Input: part model. Units: mm. Frame: model coordinates. Face numbers are marked on the shaded views. A direction names the side the tool comes from. Coordinates: 2 decimals unless noted, no trailing zeros. Write each loop counter-clockwise with the first axis right and the second up, starting at its lowest first coordinate (ties: lowest second). Pieces come first, ordered by that corner, then holes.
Autodesk Inventor part; units mm, degrees
ref_plane "YZ Plane" through (0, 0, 0) normal (1, 0, 0) x (0, 1, 0)
ref_plane "XZ Plane" through (0, 0, 0) normal (0, 1, 0) x (-1, 0, 0)
ref_plane "XY Plane" through (0, 0, 0) normal (0, 0, 1) x (1, 0, 0)
sketch "Boceto1" plane through (0, 0, 0) normal (0, 0, 1) x (1, 0, 0)
  arc A0 (30, 0) -> (-30, 0) centre (0, 0) ccw
  line L0 (5, 0) -> (30, 0)
  arc A1 (-30, 0) -> (30, 0) centre (0, 0) ccw
  circle A2 centre (0, 0) radius 5
  line L1 (0, 0) -> (0, 12.5)
  line L2 (0, 12.5) -> (-12.5, 12.5)
  line L3 (-12.5, 12.5) -> (-12.5, 16.7)
  line L4 (-12.5, 16.7) -> (12.5, 16.7)
  line L5 (12.5, 16.7) -> (12.5, 12.5)
  line L6 (12.5, 12.5) -> (0, 12.5)
  line L7 (0, 0) -> (0, -12.5)
  line L8 (0, -12.5) -> (-12.5, -12.5)
  line L9 (-12.5, -12.5) -> (-12.5, -16.7)
  line L10 (-12.5, -16.7) -> (12.5, -16.7)
  line L11 (12.5, -16.7) -> (12.5, -12.5)
  line L12 (0, -12.5) -> (12.5, -12.5)
  point P0 (0.3554, 29.9979)
  point P1 (0.3554, -29.9979)
  point P2 (-5, 0)
  dimension "d0" = 60
  dimension "d13" = 10
  dimension "d14" = 12.5
  dimension "d15" = 12.5
  dimension "d16" = 4.2
  dimension "d17" = 25
  dimension "d18" = 12.5
  dimension "d19" = 12.5
  dimension "d20" = 4.2
  dimension "d21" = 25
extrude "Extrusión2" add sketch "Boceto1" along normal blind 8
properties part number "leva00" material "Madera (abedul)"
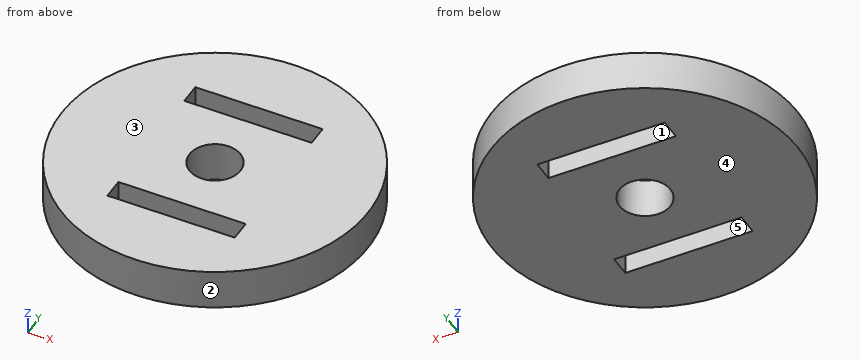
Item 1: Section query A-A, the plane x = 0. Return loops of the section in (y, z), then the cut area to 3 significant figures.
Item 2: Section query B-B, the plane z = 6.5. Return loops of the section in (x, y).
Item 3: Material intervals for line 1 (Y direction, x = 0, z = 5.5); line 2 (X direction, y = 0, z = 4.5); line 3 (Y direction, x = -9, z = 3.5), sorted ascending.
Item 4: Pin query (flat end, axial travel): pin 1 Ø2 at (y, z) = (13.5, 4.5) entering from -X; pin 2 Ø4.5 at (y, z) = (-14, 3.5) entering from +X; pin 3 Ø1 at (x, z) = (16.5, 3.5) entering from -Y. Return the tip coordinate at first contact, or that it passes through.
Item 5: Section query D-D, the plane x = 9. Return loops of the section in (y, z), then the cut area to 3 significant figures.
Item 6: Section query C-C, the plane y = 2. Return loops of the section in (x, z).
Item 7: Pull-direction query (X, two-part tool) for the marked faces 1, 2 and 3; classes: released by +X, released by -X, zero draft, split by the parting line, or undercut.
Item 8: Access query for the marked faces 4 and 5. Directions: +Z, -Z, +X, -X, +Y, -Y. A direction counts if a zero-diameter tool reaches every point of the face in a straight line with its end or side. Return the directions, or none.
The answers:
1. outline: (-30, 0) - (-16.7, 0) - (-16.7, 8) - (-30, 8) - close; (-12.5, 0) - (-5, 0) - (-5, 8) - (-12.5, 8) - close; (5, 0) - (12.5, 0) - (12.5, 8) - (5, 8) - close; (16.7, 0) - (30, 0) - (30, 8) - (16.7, 8) - close
1. area: 333 mm2
2. outline: circle Ø60 at (0, 0); hole (-12.5, -16.7) - (12.5, -16.7) - (12.5, -12.5) - (-12.5, -12.5) - close; hole (-12.5, 12.5) - (12.5, 12.5) - (12.5, 16.7) - (-12.5, 16.7) - close; hole circle Ø10 at (0, 0)
3. line 1: y = -30 to -16.7, -12.5 to -5, 5 to 12.5, 16.7 to 30
3. line 2: x = -30 to -5, 5 to 30
3. line 3: y = -28.62 to -16.7, -12.5 to 12.5, 16.7 to 28.62
4. pin 1: stops at x = -27.27
4. pin 2: stops at x = 27.6
4. pin 3: stops at y = -25.38
5. outline: (-28.62, 0) - (-16.7, 0) - (-16.7, 8) - (-28.62, 8) - close; (-12.5, 0) - (12.5, 0) - (12.5, 8) - (-12.5, 8) - close; (16.7, 0) - (28.62, 0) - (28.62, 8) - (16.7, 8) - close
5. area: 391 mm2
6. outline: (-29.93, 0) - (-4.58, 0) - (-4.58, 8) - (-29.93, 8) - close; (4.58, 0) - (29.93, 0) - (29.93, 8) - (4.58, 8) - close
7. face 1: undercut
7. face 2: split by the parting line
7. face 3: zero draft
8. face 4: -Z, +X, -X, +Y, -Y
8. face 5: +Z, -Z
